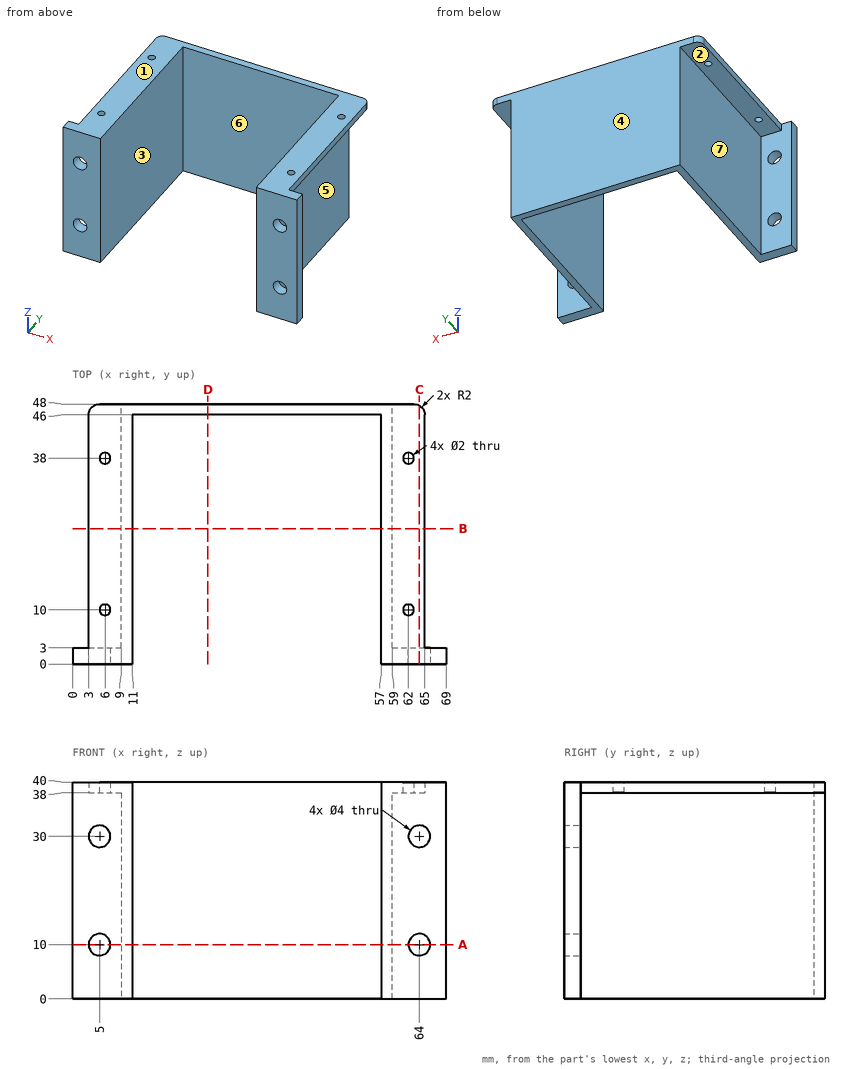
The figure shows three views and two pictorial views of one solid part (mm, origin at its lowest corner). Answer the questions. A direction names the side the tool comes from. Round coordinates to 2 decimals unless told otherwise and drop trailing zeros. Write each loop counter-clockwise with the first axis right and the second up, starting at its lowest first coordinate (ties: lowest second). Pieces come first, ordered by that corner, then holes. Notation, with made-up numbers: M -7,-19 L 41,-19 A7 cw 41,-12 Z; hole C 13,-6 d11. An arc over 180 degrees is marked long. Write each question's results on one line, items separated by ' | '. Start each with the question number.
(1) The part is cut by section C-C, the plane x = 64. Write down the section's boundary in (y, z).
(2) Each of these flat-tipped pins is pushed along its axis until it touches: P1, Ø2.5, axis at x = 6, z = 27, coming from the +Y side; P2, Ø4, axis at y = 15.5, z = 28.5, coming from the -X side; P3, Ø1, axis at y = 21.5, z = 39.5, coming from the -X side; P4, Ø12, axis at y = 5, z = 21.5, coming from the +X side. Where does it stop, or does it pass through?
(3) For the marked faces 1, 2 and 3, determine the directions among +Z, -Z, +X, -X, +Y, -Y from which every point of the face is accessible in a straight line to the end or side of a thin tool.
(4) Find the intervals of material crossed by line 1 (Y direction, x = 62, z = 39.5); line 2 (Z direction, x = 5, y = 1.75); line 3 (X direction, y = 15, z = 26.5), in increasing order.
(5) The part is cut by section A-A, the plane z = 10. Write down the section's boundary in (x, y), and give its area (3 significant figures).
(6) Determine the mould class of the marked faces 4, 5, 6 and 7 for opening direction X: +X half, -X half, draft (parallel to the pull), parting line (faces both ways), or undercut.
(7) The part is cut by section D-D, the plane x = 25. Write down the section's boundary in (y, z), and give its area (3 significant figures).
(8) The part is cut by section B-B, the plane y = 25. Write down the section's boundary in (x, z), and give its area (3 significant figures).
Worked answers:
1) outline: M 0,0 L 3,0 L 3,8 L 0,8 Z; M 0,12 L 3,12 L 3,28 L 0,28 Z; M 0,32 L 3,32 L 3,38 L 47.73,38 L 47.73,40 L 0,40 Z
2) P1: stops at y = 3 | P2: stops at x = 9 | P3: stops at x = 3 | P4: stops at x = 69
3) face 1: +Z, +X, -X, +Y, -Y | face 2: -Z, -X, +Y | face 3: +Z, -Z, -Y
4) line 1: y = 0 to 9, 11 to 37, 39 to 48 | line 2: z = 0 to 8, 12 to 28, 32 to 40 | line 3: x = 9 to 11, 57 to 59
5) outline: M 0,0 L 3,0 L 3,3 L 0,3 Z; M 7,0 L 11,0 L 11,46 L 57,46 L 57,0 L 62,0 L 62,3 L 59,3 L 59,48 L 9,48 L 9,3 L 7,3 Z; M 66,0 L 69,0 L 69,3 L 66,3 Z | area: 317 mm²
6) face 4: draft | face 5: +X half | face 6: undercut | face 7: -X half
7) outline: M 46,0 L 48,0 L 48,40 L 46,40 Z | area: 80.0 mm²
8) outline: M 3,38 L 9,38 L 9,0 L 11,0 L 11,40 L 3,40 Z; M 57,0 L 59,0 L 59,38 L 65,38 L 65,40 L 57,40 Z | area: 184 mm²
